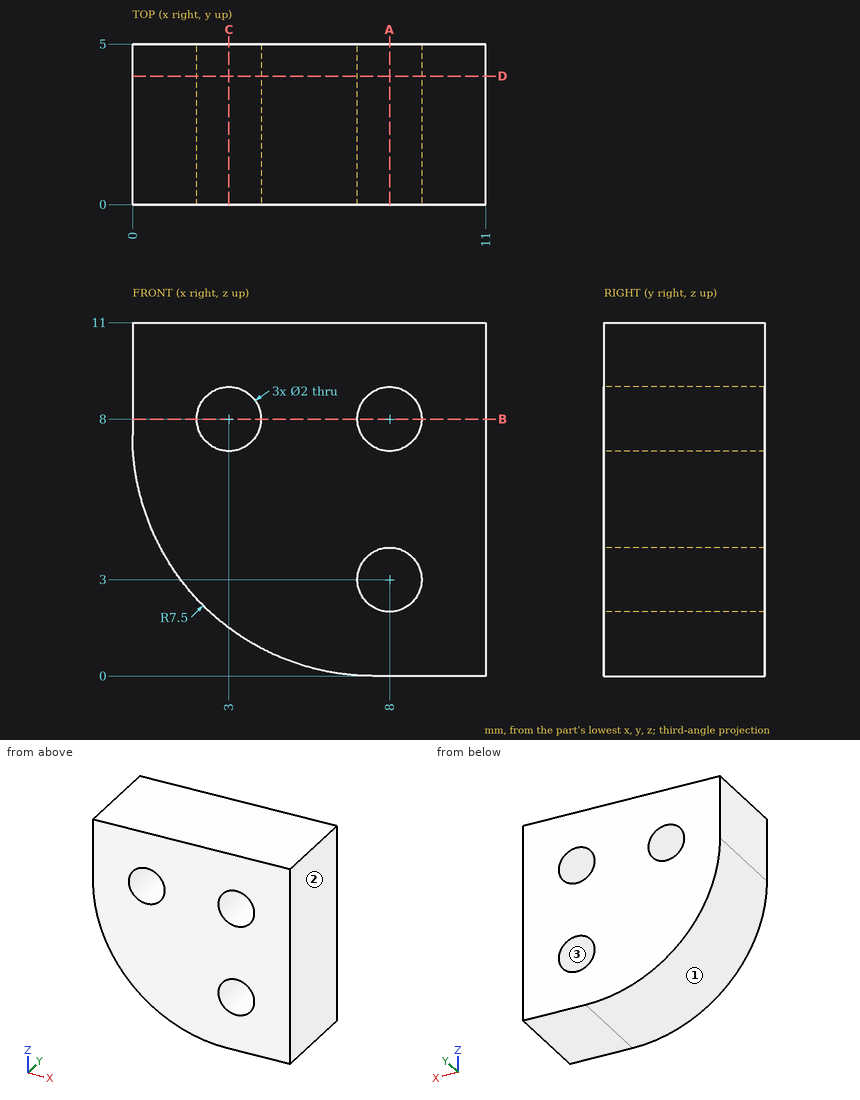
For this review, use the dimensioned drawing (mm, ordinates from the lowest corner) and the shaded views. Coordinates: 2 decimals unless noted, no trailing zeros. Loops run counter-clockwise (first coordinate to the right, second up) from the corner with the lowest first, then second, coordinate; pieces in that order, holes last.
1. Add section B-B, the plane z = 8. Give the boundary of the cut face in (x, y).
2. Insertion check: P1, Ø1.6, axis at x = 3, z = 8, coming from the +Y side; P2, Ø1.5, axis at y = 4, z = 4.5, coming from the -X side. Each pin has a flat end and moves straight along its axis. Give the tip position at first contact, or say it passes through.
3. Add section C-C, the plane x = 3. Give the boundary of the cut face in (y, z), then the cut area to 3 significant figures.
4. Add section D-D, the plane y = 4. Give the boundary of the cut face in (x, z), then the cut area to 3 significant figures.
5. Add section A-A, the plane x = 8. Give the boundary of the cut face in (y, z).
6. Mouldability with a two-part tool opening along X and no side actions: class the marked faces 1, 2 and 3 as +X half, -X half, draft (parallel to the pull), parting line (faces both ways), or undercut.
7. For line 1 (Z direction, x = 8, y = 3.85); line 2 (X direction, y = 4.7, z = 8.5); line 3 (Z direction, x = 3, y = 2.8), list the stretches that pass through material, from the lowest coordinate up.
Result:
1. outline: (0, 0) - (2, 0) - (2, 5) - (0, 5) - close; (4, 0) - (7, 0) - (7, 5) - (4, 5) - close; (9, 0) - (11, 0) - (11, 5) - (9, 5) - close
2. P1: passes through
2. P2: stops at x = 0.35
3. outline: (0, 1.5) - (5, 1.5) - (5, 7) - (0, 7) - close; (0, 9) - (5, 9) - (5, 11) - (0, 11) - close
3. area: 37.5 mm2
4. outline: (0, 7.5) arc R7.5 ccw to (7.5, 0) - (11, 0) - (11, 11) - (0, 11) - close; hole circle Ø2 at (3, 8); hole circle Ø2 at (8, 3); hole circle Ø2 at (8, 8)
4. area: 99.5 mm2
5. outline: (0, 0) - (5, 0) - (5, 2) - (0, 2) - close; (0, 4) - (5, 4) - (5, 7) - (0, 7) - close; (0, 9) - (5, 9) - (5, 11) - (0, 11) - close
6. face 1: -X half
6. face 2: +X half
6. face 3: undercut
7. line 1: z = 0 to 2, 4 to 7, 9 to 11
7. line 2: x = 0 to 2.13, 3.87 to 7.13, 8.87 to 11
7. line 3: z = 1.5 to 7, 9 to 11
